```python
from build123d import *

# Parameters (mm, degrees)
SKETCH2_W           = 150
SKETCH2_H           = 110
BOSS_EXTRUDE1_DEPTH = 3
SKETCH3_R           = 2.5
BOSS_EXTRUDE2_DEPTH = 10
SKETCH4_R           = 1.25
BOSS_EXTRUDE3_DEPTH = 5
SKETCH5_W           = 45
SKETCH5_H           = 25
CUT_EXTRUDE1_DEPTH  = 3
SKETCH6_R           = 10
CUT_EXTRUDE2_DEPTH  = 3
SKETCH7_R           = 1.2
CUT_EXTRUDE3_DEPTH  = 3


with BuildPart() as part:
    # Sketch2 → Boss-Extrude1 (new body)
    with BuildSketch(Plane(origin=(0, 0, 0), x_dir=(1, 0, 0), z_dir=(0, 1, 0))):
        Rectangle(SKETCH2_W, SKETCH2_H)
    extrude(amount=-BOSS_EXTRUDE1_DEPTH)

    # Sketch3 → Boss-Extrude2 (add)
    with BuildSketch(Plane.XZ.offset(3)):
        with Locations(Location((-17.5, 51.7, 0), (0, 0, 90))):
            Circle(SKETCH3_R)
        with Locations(Location((17.5, 51.7, 0), (0, 0, 90))):
            Circle(SKETCH3_R)
        with Locations(Location((66.25, 18, 0), (0, 0, 90))):
            Circle(SKETCH3_R)
        with Locations(Location((66.25, -22, 0), (0, 0, 90))):
            Circle(SKETCH3_R)
        with Locations(Location((-66.25, 18, 0), (0, 0, 90))):
            Circle(SKETCH3_R)
        with Locations(Location((-66.25, -22, 0), (0, 0, 90))):
            Circle(SKETCH3_R)
    extrude(amount=BOSS_EXTRUDE2_DEPTH)

    # Sketch4 → Boss-Extrude3 (add)
    with BuildSketch(Plane.XZ.offset(13)):
        with Locations(Location((17.5, 51.7, 0), (0, 0, 270))):
            Circle(SKETCH4_R)
        with Locations(Location((-17.5, 51.7, 0), (0, 0, 270))):
            Circle(SKETCH4_R)
        with Locations(Location((-66.25, 18, 0), (0, 0, 270))):
            Circle(SKETCH4_R)
        with Locations(Location((-66.25, -22, 0), (0, 0, 270))):
            Circle(SKETCH4_R)
        with Locations(Location((66.25, -22, 0), (0, 0, 270))):
            Circle(SKETCH4_R)
        with Locations(Location((66.25, 18, 0), (0, 0, 270))):
            Circle(SKETCH4_R)
    extrude(amount=BOSS_EXTRUDE3_DEPTH)

    # Sketch5 → Cut-Extrude1 (cut)
    with BuildSketch(Plane(origin=(0, 0, 0), x_dir=(1, 0, 0), z_dir=(0, 1, 0))):
        with Locations((-52.5, 2)):
            Rectangle(SKETCH5_W, SKETCH5_H)
        with Locations((52.5, 2)):
            Rectangle(SKETCH5_W, SKETCH5_H)
    extrude(amount=-CUT_EXTRUDE1_DEPTH, mode=Mode.SUBTRACT)

    # Sketch6 → Cut-Extrude2 (cut)
    with BuildSketch(Plane(origin=(0, 0, 0), x_dir=(1, 0, 0), z_dir=(0, 1, 0))):
        with Locations(Location((-32, 27, 0), (0, 0, 270))):
            Circle(SKETCH6_R)
        with Locations(Location((-32, -27, 0), (0, 0, 270))):
            Circle(SKETCH6_R)
        with Locations(Location((32, -27, 0), (0, 0, 270))):
            Circle(SKETCH6_R)
        with Locations(Location((32, 27, 0), (0, 0, 270))):
            Circle(SKETCH6_R)
    extrude(amount=-CUT_EXTRUDE2_DEPTH, mode=Mode.SUBTRACT)

    # Sketch7 → Cut-Extrude3 (cut)
    with BuildSketch(Plane(origin=(0, 0, 0), x_dir=(1, 0, 0), z_dir=(0, 1, 0))):
        with Locations(Location((-22.68, 8.95, 0), (0, 0, 270))):
            Circle(SKETCH7_R)
        with Locations(Location((22.68, 8.95, 0), (0, 0, 270))):
            Circle(SKETCH7_R)
        with Locations(Location((22.68, -8.95, 0), (0, 0, 270))):
            Circle(SKETCH7_R)
        with Locations(Location((-22.68, -8.95, 0), (0, 0, 270))):
            Circle(SKETCH7_R)
        with BuildLine():
            Line((-20.48, 11.4), (20.48, 11.4))
            Line((20.48, 11.4), (20.48, 8.95))
            ThreePointArc((20.48, 8.95), (21.124365081, 7.394365081), (22.68, 6.75))
            Line((22.68, 6.75), (25.5, 6.75))
            Line((25.5, 6.75), (25.5, -6.75))
            Line((25.5, -6.75), (22.68, -6.75))
            ThreePointArc((22.68, -6.75), (21.124365081, -7.394365081), (20.48, -8.95))
            Line((20.48, -8.95), (20.48, -11.4))
            Line((20.48, -11.4), (-20.48, -11.4))
            Line((-20.48, -11.4), (-20.48, -8.95))
            ThreePointArc((-20.48, -8.95), (-21.124365081, -7.394365081), (-22.68, -6.75))
            Line((-22.68, -6.75), (-25.5, -6.75))
            Line((-25.5, -6.75), (-25.5, 6.75))
            Line((-25.5, 6.75), (-22.68, 6.75))
            ThreePointArc((-22.68, 6.75), (-21.124365081, 7.394365081), (-20.48, 8.95))
            Line((-20.48, 8.95), (-20.48, 11.4))
        make_face()
    extrude(amount=-CUT_EXTRUDE3_DEPTH, mode=Mode.SUBTRACT)


solid = part.part
```
Design review of the part built by this model. Coordinates are the model's own, in mm. A direction names the side the tool comes from. Round coordinates to 2 decimals unless told otherwise and drop trailing zeros. Order: outer loops, then holes, each group sorted by start corner. A loop starts at its lowest first (then second) coordinate and runs counter-clockwise, first axis right, second up. Notation, with made-up numbers: (-9, -27.5) - (47, -27.5) arc R5 cw to (47, -21.5) - close; hole circle Ø9 at (51.25, 35.5). An arc over 180 degrees is marked (long way). Return JSON: item names as keys, results as strings.
Q1. Consider section C-C on z = 27. Write out the cut boundary in (x, y), plus the area to 3 significant figures.
Computed values:
{"outline": "(-75, -3) - (-42, -3) - (-42, 0) - (-75, 0) - close; (-22, -3) - (22, -3) - (22, 0) - (-22, 0) - close; (42, -3) - (75, -3) - (75, 0) - (42, 0) - close", "area": "330 mm2"}
Q2. Consider section D-D on x = -32. Write out the cut boundary in (y, z).
Computed values:
{"outline": "(-3, -55) - (0, -55) - (0, -37) - (-3, -37) - close; (-3, -17) - (0, -17) - (0, -14.5) - (-3, -14.5) - close; (-3, 10.5) - (0, 10.5) - (0, 17) - (-3, 17) - close; (-3, 37) - (0, 37) - (0, 55) - (-3, 55) - close"}
Q3. For pin 1 Ø6 at (y, z) = (-4, 37) entering from +X; pin 2 Ø1.2 at (y, z) = (-1, 9.5) entering from +X; pin 3 Ø2 at (x, z) = (31.5, -15) entering from -Y, all flat-tipped, find the tip position at first contact; note any pin that passes through.
Computed values:
{"pin 1": "stops at x = 75", "pin 2": "stops at x = 30", "pin 3": "stops at y = -3"}
Q4. Consider section B-B on x = -52.5. Write out the cut boundary in (y, z), plus the area to 3 significant figures.
Computed values:
{"outline": "(-3, -55) - (0, -55) - (0, -14.5) - (-3, -14.5) - close; (-3, 10.5) - (0, 10.5) - (0, 55) - (-3, 55) - close", "area": "255 mm2"}
Q5. The part is to be moulded in two halves that separate along X. For faces 4 (the flat face through (30, -1, -2)), 5 (the cylindrical face through (-66.36, -7.93, -24.498)), 6 (the flat face through (-75, -1, -34)), 7 (the flat face through (52, -1, 10.5)), say which applies: pulls with the +X half, pulls with the -X half, needs draft (parallel to the pull), parting line crosses it, or undercut.
Computed values:
{"face 4": "pulls with the +X half", "face 5": "undercut", "face 6": "pulls with the -X half", "face 7": "needs draft"}
Q6. Machinability: for faces 1 (the flat face through (24, -1, 6.75)), 2 (the cylindrical face through (66.14, -7.93, -24.498)), 3 (the flat face through (52, -1, -14.5)), which of the approach directions +Z, -Z, +X, -X, +Y, -Y give a long, thin tool a straight path to every point of the face, cutting with its end or side? Answer none if there is none.
Computed values:
{"face 1": "+Y, -Y", "face 2": "-Y", "face 3": "+X, +Y, -Y"}
Q7. Consider section A-A on y = -15. Write out the cut boundary in (x, z), plus the area to 3 significant figures.
Computed values:
{"outline": "circle Ø2.5 at (-66.25, -22); circle Ø2.5 at (-66.25, 18); circle Ø2.5 at (-17.5, 51.7); circle Ø2.5 at (17.5, 51.7); circle Ø2.5 at (66.25, -22); circle Ø2.5 at (66.25, 18)", "area": "29.5 mm2"}
Q8. Wall thickness on L1, parallel to X at y = -2.1, z = 27; L2, parallel to Z at x = 17.5, y = -1.5; L3, parallel to X at y = -1.5, z = -6: over which ranges is each line inside the solid? List them lowest first. Write a range as [from, to].
Computed values:
{"L1": "x = [-75, -42], [-22, 22], [42, 75]", "L2": "z = [-55, -11.4], [11.4, 55]", "L3": "x = [-30, -25.5], [25.5, 30]"}
